Could you check a few things on this model? Use its own coordinates, in mm. A direction names the side the tool comes from. Give positions to 0.01 mm unless a question says otherwise; leave off trailing zeros. Write each loop counter-clockwise with the first axis right and the second up, starting at its lowest first coordinate (ties: lowest second). Pieces come first, ordered by that corner, then holes. Notation, with made-up numbers: (39, 27) -> (43, 27) arc R29 cw to (43, 47) -> close; hole circle Ø6 at (38.5, 6). An arc over 180 degrees is marked (long way). Write item = value, one per line. Start each with the question number.
```python
from build123d import *

# Parameters (mm, degrees)
SKETCH1_W           = 121.5
SKETCH1_H           = 125
BOSS_EXTRUDE1_DEPTH = 2.4
BOSS_EXTRUDE2_DEPTH = 125
SKETCH4_R           = 1.7
CUT_EXTRUDE1_DEPTH  = 92.401490688
CUT_EXTRUDE2_DEPTH  = 92.401490688
SKETCH6_R           = 1.7
CUT_EXTRUDE3_DEPTH  = 92.401490688
CUT_EXTRUDE4_DEPTH  = 92.401490688
CIRPATTERN1_COUNT   = 4


with BuildPart() as part:
    # Sketch1 → Boss-Extrude1 (new body)
    with BuildSketch(Plane(origin=(0, 0, 0), x_dir=(1, 0, 0), z_dir=(0, 1, 0))):
        Rectangle(SKETCH1_W, SKETCH1_H)
    extrude(amount=BOSS_EXTRUDE1_DEPTH)

    # Sketch3 → Boss-Extrude2 (add)
    with BuildSketch(Plane.XY.offset(62.5)):
        Polygon((60.75, 0), (60.75, 2.4), (62.55, 2.4), (62.65, 2.4), (62.65, 4.61), (64.508602565, 4.61), (66.65, 2.470350907), (66.65, 0), align=None)
    extrude(amount=-BOSS_EXTRUDE2_DEPTH)

    # Sketch4 → Cut-Extrude1 (cut, through all)
    with BuildSketch(Plane(origin=(0, 2.4, 0), x_dir=(1, 0, 0), z_dir=(0, 1, 0))):
        with Locations(Location((57.25, -59, 0), (0, 0, 270))):
            Circle(SKETCH4_R)
    extrude(amount=-CUT_EXTRUDE1_DEPTH, mode=Mode.SUBTRACT)

    # Sketch5 → Cut-Extrude2 (cut, through all)
    with BuildSketch(Plane(origin=(0, 2.4, 0), x_dir=(1, 0, 0), z_dir=(0, 1, 0))):
        with BuildLine():
            Line((58.25, 47.5), (58.25, 62.5))
            Line((58.25, 62.5), (48.25, 62.5))
            Line((48.25, 62.5), (48.25, 47.5))
            ThreePointArc((48.25, 47.5), (53.25, 42.5), (58.25, 47.5))
        make_face()
    extrude(amount=-CUT_EXTRUDE2_DEPTH, mode=Mode.SUBTRACT)

    # Sketch6 → Cut-Extrude3 (cut, through all)
    with BuildSketch(Plane(origin=(0, 2.4, 0), x_dir=(1, 0, 0), z_dir=(0, 1, 0))):
        with Locations(Location((-1.25, -23.5, 0), (0, 0, 270))):
            Circle(SKETCH6_R)
        with Locations(Location((30.75, -23.5, 0), (0, 0, 270))):
            Circle(SKETCH6_R)
        with Locations(Location((30.75, 8.5, 0), (0, 0, 270))):
            Circle(SKETCH6_R)
        with Locations(Location((-1.25, 8.5, 0), (0, 0, 270))):
            Circle(SKETCH6_R)
    extrude(amount=-CUT_EXTRUDE3_DEPTH, mode=Mode.SUBTRACT)

    # Sketch7 → Cut-Extrude4 (cut, through all)
    with BuildSketch(Plane(origin=(0, 2.4, 0), x_dir=(1, 0, 0), z_dir=(0, 1, 0))):
        with BuildLine():
            Line((15.256250977, -7), (20.900523404, -7))
            ThreePointArc((20.900523404, -7), (19.115269425, -3.140981552), (15.256250977, -1.355727573))
            Line((15.256250977, -1.355727573), (15.256250977, -7))
        make_face()
        with BuildLine():
            Line((21.903365757, -7), (27.575669866, -7))
            ThreePointArc((27.575669866, -7), (23.827841263, 1.571590286), (15.256250977, 5.319418889))
            Line((15.256250977, 5.319418889), (15.256250977, -0.35288522))
            ThreePointArc((15.256250977, -0.35288522), (19.822376206, -2.433874771), (21.903365757, -7))
        make_face()
        with BuildLine():
            ThreePointArc((15.256250977, 6.320124192), (24.534948045, 2.278697068), (28.576375169, -7))
            Line((28.576375169, -7), (34.75, -7))
            ThreePointArc((34.75, -7), (28.898386601, 6.642135624), (15.256250977, 12.493749023))
            Line((15.256250977, 12.493749023), (15.256250977, 6.320124192))
        make_face()
    cut_extrude4 = extrude(amount=-CUT_EXTRUDE4_DEPTH, mode=Mode.SUBTRACT)

    # CirPattern1: Cut-Extrude4 ×4 about axis
    cirpattern1_axis = Axis((14.756250977, 0, 7.5), (0, 1, 0))
    for i in range(1, CIRPATTERN1_COUNT):
        add(cut_extrude4.rotate(cirpattern1_axis, i * 360 / CIRPATTERN1_COUNT), mode=Mode.SUBTRACT)


solid = part.part
```
(1) On a 3-axis mill with a long thin cutter (end or side, diameter ignored), from which of +Z, -Z, +X, -X, +Y, -Y can I reach the whole of each face in a straight line? I mean faces 1 (the cylindrical face through (28.75, 1.22, 21.79)), 2 (the cylindrical face through (53.14, 1.22, -42.5)). Say none if no direction works.
(2) Imagine slicing it at B-B (z = -8.5). Please give me the cut outline in (x, y), then the cut area to 3 significant figures.
(3) We'd pull the mould along X, two halves only. Please class faces 3 (the cylindrical face through (23.7, 1.2, 16.7)), 4 (the flat face through (-10, 0, 1)): released by +X, released by -X, zero draft, split by the parting line, or undercut.
(4) Imagine slicing it at A-A (z = -53.5). Please give me the cut outline in (x, y), then the cut area to 3 significant figures.
(5) I'm going to push a flat-ended pin straight in: pin 1 (2 mm diameter, centred on x = -42, z = 14, fed in from +Y). Where does the tip first touch, or does it pass through?
(6) Imagine slicing it at C-C (x = 30.75). Please give me the cut outline in (y, z), then the cut area to 3 significant figures.
(7) If I drill on line 1 along X through (y, z) = (1.2, 23.5); line 2 along Z through (x, y) = (25.5, 0.45); line 3 along Y through (x, z) = (-30, -21), over which ranges is the centre line in solid material (lowest first)? Write a range as from..to.
(8) Imagine slicing it at D-D (y = 1.4). State how many separate pieces and enclosed holes the cut face has, then the cut area to 3 significant figures.
Answers below:
q1.face_1 = +Y, -Y
q1.face_2 = -Z, +Y, -Y
q2.outline = (-60.75, 0) -> (-2.95, 0) -> (-2.95, 2.4) -> (-60.75, 2.4) -> close; (0.45, 0) -> (2.76, 0) -> (2.76, 2.4) -> (0.45, 2.4) -> close; (14.26, 0) -> (15.26, 0) -> (15.26, 2.4) -> (14.26, 2.4) -> close; (26.76, 0) -> (29.05, 0) -> (29.05, 2.4) -> (26.76, 2.4) -> close; (32.45, 0) -> (66.65, 0) -> (66.65, 2.47) -> (64.51, 4.61) -> (62.65, 4.61) -> (62.65, 2.4) -> (32.45, 2.4) -> close
q2.area = 241 mm^2
q3.face_3 = undercut
q3.face_4 = zero draft
q4.outline = (-60.75, 0) -> (48.25, 0) -> (48.25, 2.4) -> (-60.75, 2.4) -> close; (58.25, 0) -> (66.65, 0) -> (66.65, 2.47) -> (64.51, 4.61) -> (62.65, 4.61) -> (62.65, 2.4) -> (58.25, 2.4) -> close
q4.area = 288 mm^2
q5.pin_1 = 2.4
q6.outline = (0, -62.5) -> (2.4, -62.5) -> (2.4, -10.2) -> (0, -10.2) -> close; (0, -6.8) -> (2.4, -6.8) -> (2.4, -4.51) -> (0, -4.51) -> close; (0, 7) -> (2.4, 7) -> (2.4, 8) -> (0, 8) -> close; (0, 19.51) -> (2.4, 19.51) -> (2.4, 21.8) -> (0, 21.8) -> close; (0, 25.2) -> (2.4, 25.2) -> (2.4, 62.5) -> (0, 62.5) -> close
q6.area = 228 mm^2
q7.line_1 = -60.75..-2.95, 0.45..2.76, 14.26..15.26, 26.76..29.05, 32.45..66.65
q7.line_2 = -62.5..-9.37, -1.21..0.49, 7..8, 14.51..16.21, 24.37..62.5
q7.line_3 = 0..2.4
q8.separate_pieces = 1
q8.enclosed_holes = 17
q8.area = 14,600 mm^2
